Study the drawing (mm; zero at the part's minimum x, y, z) and answer. Give positions to 0.01 mm unless a question says otherwise; leave off trailing zeros. Write each loop counter-clockwise with the first axis right and the second up, starting at its lowest first coordinate (ties: lowest second). Pieces come first, ordered by that corner, then holes. Notation, with made-up numbers: M 20,-37 L 34,-37 A23 ccw 34,-8 Z; hole C 48.25,26.25 d11. An arc over 180 degrees is marked long. Use a Markdown table: item, result. Add a question column.
Item 1: Given P1, Ø2.5, axis at x = 9.975, y = 16.975, coming from the +Z side; P2, Ø8, axis at x = 9.975, y = 9.975, coming from the -Z side, each flat-ended and moving along its own axis, determine where each tip first touches the part or whether it passes through.
Item 2: The mould has two halves that part along Y. Classify the marked faces 1, 2, 3 and 4: pulls with the +Y half, pulls with the -Y half, needs draft (parallel to the pull), parting line crosses it, or undercut.
Item 3: A cutting plane is placed at D-D on z = 2.6. Determine the outline of the cut face in (x, y) (3 decimals).
Item 4: A cutting plane is placed at A-A on y = 9.5. Determine the outline of the cut face in (x, z), then the cut area to 3 significant figures.
Item 5: A cutting plane is placed at C-C on y = 17. Determine the outline of the cut face in (x, z).
Item 6: A cutting plane is placed at B-B on x = 7.75. Determine the outline of the cut face in (y, z).
Item 7: Consider probe 1 along X at (y, z) = (2.25, 2.05); probe 2 along X at (y, z) = (2.5, 2.65). Determine where each line is inside the solid, lowest interval first. Write a range as [from, to].
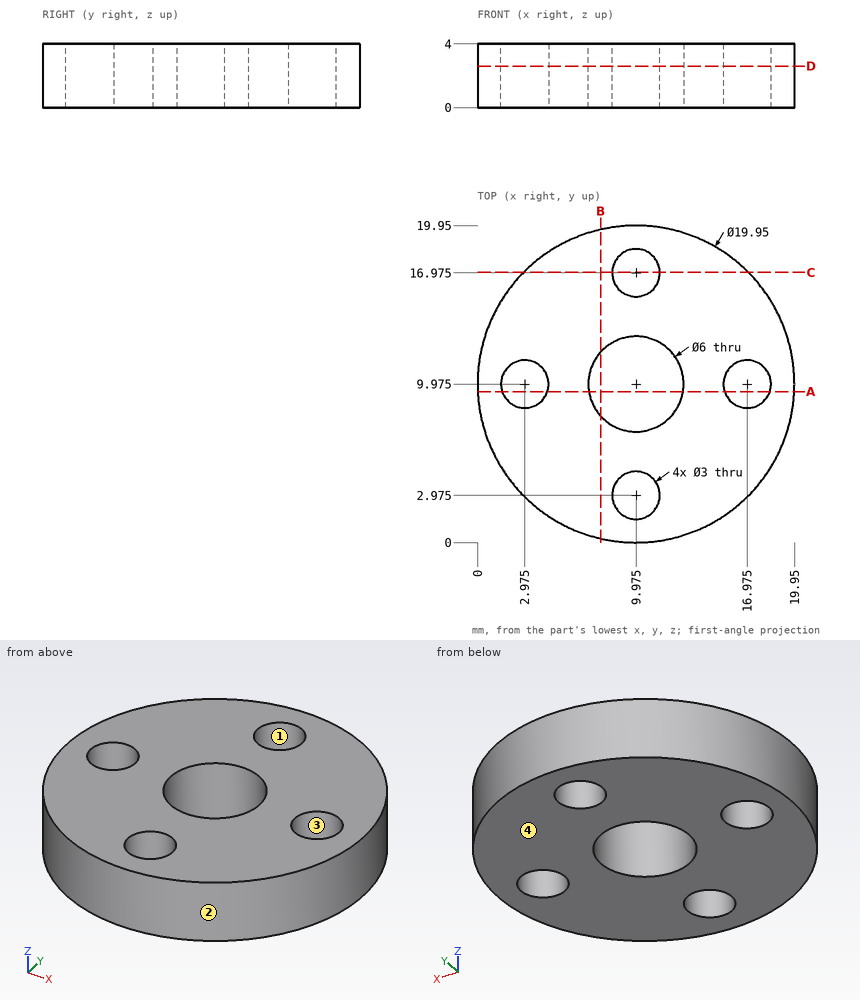
Filled in:
| question | item | result |
|---|---|---|
| 1 | P1 | through |
| 1 | P2 | z = 0 |
| 2 | face 1 | undercut |
| 2 | face 2 | parting line crosses it |
| 2 | face 3 | undercut |
| 2 | face 4 | needs draft |
| 3 | outline | C 9.975,9.975 d19.95; hole C 2.975,9.975 d3; hole C 9.975,9.975 d6; hole C 9.975,2.975 d3; hole C 9.975,16.975 d3; hole C 16.975,9.975 d3 |
| 4 | outline | M 0.01,0 L 1.55,0 L 1.55,4 L 0.01,4 Z; M 4.4,0 L 7.01,0 L 7.01,4 L 4.4,4 Z; M 12.94,0 L 15.55,0 L 15.55,4 L 12.94,4 Z; M 18.4,0 L 19.94,0 L 19.94,4 L 18.4,4 Z |
| 4 | area | 33.2 mm² |
| 5 | outline | M 2.89,0 L 8.48,0 L 8.48,4 L 2.89,4 Z; M 11.47,0 L 17.06,0 L 17.06,4 L 11.47,4 Z |
| 6 | outline | M 0.25,0 L 7.96,0 L 7.96,4 L 0.25,4 Z; M 11.99,0 L 19.7,0 L 19.7,4 L 11.99,4 Z |
| 7 | probe 1 | [3.66, 8.66], [11.29, 16.29] |
| 7 | probe 2 | [3.37, 8.55], [11.4, 16.58] |
